Autodesk Fusion 360 part; units mm, degrees
sketch "Sketch1" plane through (0, 0, 0) normal (0, 0, 1) x (1, 0, 0)
  circle A0 centre (0, 0) radius 11
  circle A1 centre (0, 0) radius 4
  dimension "d1" = 22
  dimension "d2" = 8
extrude "Extrude1" add sketch "Sketch1" along normal blind 7
fillet "Fillet1" radius 0.75 2 edges at (-10.2556, -3.9778, 7) (-10.2556, -3.9778, 0)
fillet "Fillet2" radius 0.5 2 edges at (-3.7293, 1.4465, 7) (-3.7293, 1.4465, 0)
The model under review builds one solid part; all positions refer to its coordinate system, in mm. Round coordinates to 2 decimals unless told otherwise and drop trailing zeros. Write each loop counter-clockwise with the first axis right and the second up, starting at its lowest first coordinate (ties: lowest second). Pieces come first, ordered by that corner, then holes.
(1) Mouldability with a two-part tool opening along Y and no side actions: class faces 1 (the cylindrical face through (-0.867, 3.905, 3.458)), 2 (the cylindrical face through (-2.38, 10.74, 3.46)), 3 (the flat face through (4.4, -2.1, 0)) as +Y half, -Y half, draft (parallel to the pull), parting line (faces both ways), or undercut.
(2) Wall thickness on L1, parallel to Y at x = 0, z = 2.5; L2, parallel to Y at x = -0.75, z = 5; L3, parallel to X at y = -3.5, z = 4.5: over which ranges is each line inside the solid? List them lowest first.
(3) Insertion check: pin 1 (4 mm diameter, centred on x = -4, z = 5, fed in from +Y); pin 2 (1.5 mm diameter, centred on y = 8, z = 3, fed in from -X); pin 3 (7 mm diameter, centred on x = 0, y = 0, fed in from -Z); pin 4 (4 mm diameter, centred on y = -7.5, z = 3, fed in from +X). Each pin has a flat end and moves straight along its axis. Give the tip position at first contact, or say it passes through.
(4) We need section A-A on y = 0. Give the boundary of the cut face in (x, z).
(5) We need section C-C on z = 4. Give the boundary of the cut face in (x, y), and give its area (3 significant figures).
Findings below:
1. face 1: undercut
1. face 2: parting line
1. face 3: draft
2. L1: y = -11 to -4, 4 to 11
2. L2: y = -10.97 to -3.93, 3.93 to 10.97
2. L3: x = -10.43 to -1.94, 1.94 to 10.43
3. pin 1: stops at y = 10.82
3. pin 2: stops at x = -8.27
3. pin 3: passes through
3. pin 4: stops at x = 9.53
4. outline: (-11, 0.75) arc R0.75 ccw to (-10.25, 0) - (-4.5, 0) arc R0.5 ccw to (-4, 0.5) - (-4, 6.5) arc R0.5 ccw to (-4.5, 7) - (-10.25, 7) arc R0.75 ccw to (-11, 6.25) - close; (4, 0.5) arc R0.5 ccw to (4.5, 0) - (10.25, 0) arc R0.75 ccw to (11, 0.75) - (11, 6.25) arc R0.75 ccw to (10.25, 7) - (4.5, 7) arc R0.5 ccw to (4, 6.5) - close
5. outline: circle Ø22 at (0, 0); hole circle Ø8 at (0, 0)
5. area: 330 mm2
